```python
from build123d import *

# Parameters (mm, degrees)
SKETCH_W     = 247
SKETCH_H     = 150
PAD_DEPTH    = 18
POCKET_DEPTH = 18.001
CHAMFER_SIZE = 9


with BuildPart() as part:
    # Sketch → Pad (new body)
    with BuildSketch(Plane.XY):
        with Locations((-123.5, 75)):
            Rectangle(SKETCH_W, SKETCH_H)
    extrude(amount=PAD_DEPTH)

    # Sketch001 (on Face6 of Pad) → Pocket (cut, through all)
    with BuildSketch(Plane.XY.offset(18)):
        with BuildLine():
            ThreePointArc((-101.5, 75), (-123.5, 97), (-145.5, 75))
            Line((-145.5, 75), (-145.5, 0))
            Line((-101.5, 0), (-145.5, 0))
            Line((-101.5, 75), (-101.5, 0))
        make_face()
    extrude(amount=-POCKET_DEPTH, mode=Mode.SUBTRACT)

    # Chamfer
    chamfer_edges = [part.edges().sort_by_distance(p)[0] for p in [
        (-145.5, 37.5, 18),
        (-123.5, 97, 18),
        (-101.5, 37.5, 18),
    ]]
    chamfer(chamfer_edges, length=CHAMFER_SIZE)


solid = part.part
```
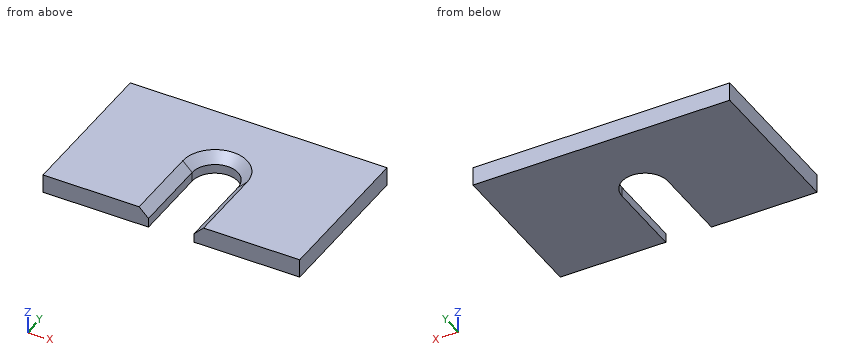
Geometry check sheet. Reference: the model listing, model coordinates, mm. Coordinates: 2 decimals unless noted, no trailing zeros. Order: outer loops, then holes, each group sorted by start corner. A loop starts at its lowest first (then second) coordinate and runs counter-clockwise, first axis right, second up. Notation, with made-up numbers: (-4.5, -3.5) - (46.5, -3.5) arc R20 cw to (46.5, 16.5) - close; hole circle Ø5 at (53, 65). An arc over 180 degrees is marked (long way). Answer as a JSON object with one key per item and string values. Group by question number.
Item 1: Scan lines: probe 1 along X at (y, z) = (29.5, 7.5); probe 2 along X at (y, z) = (19, 16.5); probe 3 along Y at (x, z) = (-118.5, 1.75). Record each from-to range of solid material in increasing order.
Item 2: Sectioned sample at A-A, the plane y = 40. Record the cut outline in (x, z), and give its area (3 significant figures).
Item 3: Sectioned sample at C-C, the plane x = -123.5. Record the cut outline in (y, z).
Item 4: Sectioned sample at B-B, the plane z = 4. Record the cut outline in (x, y).
Resolved:
{
 "1": {"probe 1": "-247 to -145.5, -101.5 to 0", "probe 2": "-247 to -153, -94 to 0", "probe 3": "96.42 to 150"},
 "2": {"outline": "(-247, 0) - (-145.5, 0) - (-145.5, 9) - (-154.5, 18) - (-247, 18) - close; (-101.5, 0) - (0, 0) - (0, 18) - (-92.5, 18) - (-101.5, 9) - close", "area": "3,570 mm^2"},
 "3": {"outline": "(97, 0) - (150, 0) - (150, 18) - (106, 18) - (97, 9) - close"},
 "4": {"outline": "(-247, 0) - (-145.5, 0) - (-145.5, 75) arc R22 cw to (-101.5, 75) - (-101.5, 0) - (0, 0) - (0, 150) - (-247, 150) - close"}
}
